Source: CAD feature listing. Evaluate the final solid. Frame: model axes, mm. A direction names the side the tool comes from. Give positions to 0.01 mm unless a question says otherwise; leave off trailing zeros. Write each loop counter-clockwise with the first axis right and the second up, starting at its lowest first coordinate (ties: lowest second). Pieces come first, ordered by that corner, then holes. Notation, with made-up numbers: (26.25, 65.25) - (30.25, 65.25) arc R31 ccw to (30.25, 101.25) - close; hole circle Ø2 at (-20.5, 35). An arc over 180 degrees is marked (long way). Answer as a JSON object with one key per item and string values. Group by question number.
from build123d import *
from build123d.topology import SkipClean

# Parameters (mm, degrees)
SKETCH1_R                = 5.5
SKETCH1_R_2              = 4.85
BOSS_EXTRUDE1_DEPTH      = 17
BOSS_EXTRUDE2_START      = -1.75
BOSS_EXTRUDE2_DEPTH      = 1.75
BOSS_EXTRUDE3_DEPTH      = 1.7
BOSS_EXTRUDE3_2_DEPTH    = 1.7
BOSS_EXTRUDE4_REACH      = 128.36
BOSS_EXTRUDE4_END_RADIUS = 4.85
SKETCH3_W                = 1.7
SKETCH3_H                = 0.6
BOSS_EXTRUDE5_START      = -9.624935
SKETCH3_2_W              = 1.7
SKETCH3_2_H              = 0.6
BOSS_EXTRUDE5_DEPTH      = 0.075066
FILLET1_R                = 0.2
BOSS_EXTRUDE6_START      = 17
SKETCH1_4_R              = 5.5
SKETCH1_4_W              = 6
SKETCH1_4_H              = 6
BOSS_EXTRUDE6_DEPTH      = 2


with BuildPart() as part:
    # Sketch1 → Boss-Extrude1 (new body)
    with BuildSketch(Plane.XZ.offset(-123.994845224)):
        with Locations(Location((0, 0, 0), (0, 0, 270))):
            Circle(SKETCH1_R)
        with Locations(Location((0, 0, 0), (0, 0, 270))):
            Circle(SKETCH1_R_2, mode=Mode.SUBTRACT)
    extrude(amount=BOSS_EXTRUDE1_DEPTH)

    # Sketch1<3> → Boss-Extrude2 (add)
    with SkipClean():  # the faces are left unmerged after this step: merging them gives an invalid solid
        with BuildSketch(Plane.XZ.offset(-123.994845224).offset(BOSS_EXTRUDE2_START)):
            with BuildLine():
                ThreePointArc((4.280924301, -3.453069233), (4.763148058, -2.74998556), (5.130919838, -1.98082347))
                Line((5.130919838, -1.98082347), (5.108754465, -1.968026376))
                Line((5.108754465, -1.968026376), (4.625228328, -1.688864385))
                Line((4.625228328, -1.688864385), (4.20023564, -2.424978467))
                Line((4.20023564, -2.424978467), (3.775232792, -3.161110148))
                Line((3.775232792, -3.161110148), (4.258758928, -3.440272139))
                Line((4.258758928, -3.440272139), (4.280924301, -3.453069233))
            make_face()
            with BuildLine():
                Line((-3.775232792, 3.161110148), (-4.258758928, 3.440272139))
                Line((-4.258758928, 3.440272139), (-4.280924301, 3.453069233))
                ThreePointArc((-4.280924301, 3.453069233), (-4.763148058, 2.74998556), (-5.130919838, 1.98082347))
                Line((-5.130919838, 1.98082347), (-5.108754465, 1.968026376))
                Line((-5.108754465, 1.968026376), (-4.625228328, 1.688864385))
                Line((-4.625228328, 1.688864385), (-4.200235262, 2.424979122))
                Line((-4.200235262, 2.424979122), (-3.775232792, 3.161110148))
            make_face()
            with BuildLine():
                Line((4.625228328, -1.688864385), (4.560219632, -1.651331859))
                ThreePointArc((4.560219632, -1.651331859), (4.397274885, -2.046087385), (4.20023564, -2.424978467))
                Line((4.20023564, -2.424978467), (4.625228328, -1.688864385))
            make_face()
            with BuildLine():
                ThreePointArc((4.20023564, -2.424978467), (3.970623818, -2.785075672), (3.710224095, -3.123577623))
                Line((3.710224095, -3.123577623), (3.775232792, -3.161110148))
                Line((3.775232792, -3.161110148), (4.20023564, -2.424978467))
            make_face()
            with BuildLine():
                ThreePointArc((-4.560219632, 1.651331859), (-4.397274725, 2.046087728), (-4.200235262, 2.424979122))
                Line((-4.200235262, 2.424979122), (-4.625228328, 1.688864385))
                Line((-4.625228328, 1.688864385), (-4.560219632, 1.651331859))
            make_face()
            with BuildLine():
                Line((-3.710224095, 3.123577623), (-3.775232792, 3.161110148))
                Line((-3.775232792, 3.161110148), (-4.200235262, 2.424979122))
                ThreePointArc((-4.200235262, 2.424979122), (-3.970623601, 2.785075982), (-3.710224095, 3.123577623))
            make_face()
        extrude(amount=BOSS_EXTRUDE2_DEPTH)



with BuildPart() as body_2:
    # Sketch2 → Boss-Extrude3 (new body)
    with BuildSketch(Plane(origin=(0.424997768, 0, 0.736122882), x_dir=(0.866026919582721, 0, -0.49999737455117027), z_dir=(0.49999737455117027, 0, 0.866026919582721))):
        Polygon((4.5, 125.144845224), (4.774934555, 125.144845224), (4.774934555, 125.744845224), align=None)
    extrude(amount=-BOSS_EXTRUDE3_DEPTH)


with BuildPart() as body_3:
    # Sketch2 → Boss-Extrude3 2 (new body)
    with BuildSketch(Plane(origin=(0.424997768, 0, 0.736122882), x_dir=(0.866026919582721, 0, -0.49999737455117027), z_dir=(0.49999737455117027, 0, 0.866026919582721))):
        Polygon((-4.5, 125.144845224), (-4.774934555, 125.744845224), (-4.774934555, 125.144845224), align=None)
    extrude(amount=-BOSS_EXTRUDE3_2_DEPTH)


with BuildPart() as part_1:
    with SkipClean():  # the faces are left unmerged after this step: merging them gives an invalid solid
        add(part.part)

        add(body_2.part)  # Boss-Extrude4 merges body 2
        # Boss-Extrude4: up to this cylinder (the profile starts inside it)
        boss_extrude4_end = Plane(origin=(0, 125.444845, 0), z_dir=(0, 1, 0)) * Cylinder(BOSS_EXTRUDE4_END_RADIUS, 267.42, mode=Mode.PRIVATE)
        # Sketch3 → Boss-Extrude4 (add, up to the surface)
        with BuildSketch(Plane(origin=(4.135221863, 0, -2.387454741), x_dir=(-0.4999973745511703, 0, -0.866026919582721), z_dir=(0.866026919582721, 0, -0.4999973745511703)), mode=Mode.PRIVATE) as boss_extrude4_sk1:
            with Locations((0, 125.444845224)):
                Rectangle(SKETCH3_W, SKETCH3_H)
        boss_extrude4_tool1 = extrude(boss_extrude4_sk1.sketch, amount=BOSS_EXTRUDE4_REACH, mode=Mode.PRIVATE) & boss_extrude4_end
        add(boss_extrude4_tool1.solids().sort_by_distance((4.135222, 125.444845, -2.387455))[0])


    with SkipClean():  # the faces are left unmerged after this step: merging them gives an invalid solid
        add(body_3.part)  # Boss-Extrude5 merges body 3
        # Sketch3<2> → Boss-Extrude5 (add)
        with BuildSketch(Plane(origin=(4.135221863, 0, -2.387454741), x_dir=(-0.4999973745511703, 0, -0.866026919582721), z_dir=(0.866026919582721, 0, -0.4999973745511703)).offset(BOSS_EXTRUDE5_START)):
            with Locations((0, 125.444845224)):
                Rectangle(SKETCH3_2_W, SKETCH3_2_H)
        extrude(amount=BOSS_EXTRUDE5_DEPTH)

    # Fillet1
    # the kernel refuses this fillet: 0.2 mm, written as the material it adds along each edge
    with BuildSketch(Plane(origin=(-4.713937761, 123.994845224, 3.70306792), x_dir=(0.49999737455195337, 0, 0.866026919582269), z_dir=(0.866026919582269, 0, -0.4999973745519534))) as fillet1_piece_1_section:
        with BuildLine():
            CenterArc((FILLET1_R, -FILLET1_R), FILLET1_R, 90, 90)
            Line((0, -FILLET1_R), (0, 0))
            Line((0, 0), (FILLET1_R, 0))
        make_face()
    fillet1_piece_1 = extrude(amount=1.083921236, mode=Mode.PRIVATE)
    fillet1_piece_1 = fillet1_piece_1 & Plane(origin=(0, 124.040443489, 0), x_dir=(0, 0, -1), z_dir=(0, 1, 0)) * Cylinder(5.5, 3, mode=Mode.PRIVATE)
    add(fillet1_piece_1)
    with BuildSketch(Plane(origin=(4.713937761, 123.994845224, -3.70306792), x_dir=(-0.49999737455261106, 0, -0.8660269195818893), z_dir=(-0.8660269195818893, 0, 0.4999973745526111))) as fillet1_piece_2_section:
        with BuildLine():
            CenterArc((FILLET1_R, -FILLET1_R), FILLET1_R, 90, 90)
            Line((0, -FILLET1_R), (0, 0))
            Line((0, 0), (FILLET1_R, 0))
        make_face()
    fillet1_piece_2 = extrude(amount=1.083921236, mode=Mode.PRIVATE)
    fillet1_piece_2 = fillet1_piece_2 & Plane(origin=(0, 124.040443489, 0), x_dir=(0, 0, -1), z_dir=(0, 1, 0)) * Cylinder(5.5, 3, mode=Mode.PRIVATE)
    add(fillet1_piece_2)
    with BuildSketch(Plane(origin=(-4.625228328, 123.994845224, 1.688864385), x_dir=(-0.49999737454985904, 0, -0.866026919583478), z_dir=(-0.8660269195834781, 0, 0.49999737454985904))) as fillet1_piece_3_section:
        with BuildLine():
            CenterArc((FILLET1_R, -FILLET1_R), FILLET1_R, 90, 90)
            Line((0, -FILLET1_R), (0, 0))
            Line((0, 0), (FILLET1_R, 0))
        make_face()
    fillet1_piece_3 = extrude(amount=1.083921236, mode=Mode.PRIVATE)
    fillet1_piece_3 = fillet1_piece_3 & Plane(origin=(0, 124.040443489, 0), x_dir=(0, 0, -1), z_dir=(0, 1, 0)) * Cylinder(5.5, 3, mode=Mode.PRIVATE)
    add(fillet1_piece_3)
    with BuildSketch(Plane(origin=(4.625228328, 123.994845224, -1.688864385), x_dir=(0.4999973745501742, 0, 0.866026919583296), z_dir=(0.8660269195832961, 0, -0.49999737455017423))) as fillet1_piece_4_section:
        with BuildLine():
            CenterArc((FILLET1_R, -FILLET1_R), FILLET1_R, 90, 90)
            Line((0, -FILLET1_R), (0, 0))
            Line((0, 0), (FILLET1_R, 0))
        make_face()
    fillet1_piece_4 = extrude(amount=1.083921236, mode=Mode.PRIVATE)
    fillet1_piece_4 = fillet1_piece_4 & Plane(origin=(0, 124.040443489, 0), x_dir=(0, 0, -1), z_dir=(0, 1, 0)) * Cylinder(5.5, 3, mode=Mode.PRIVATE)
    add(fillet1_piece_4)
    with BuildSketch(Plane(origin=(4.625228328, 123.994845224, -1.688864385), x_dir=(0.4999973745511805, 0, 0.8660269195827152), z_dir=(-0.8660269195827152, 0, 0.49999737455118054))) as fillet1_piece_5_section:
        with BuildLine():
            CenterArc((FILLET1_R, FILLET1_R), FILLET1_R, 180, 90)
            Line((0, FILLET1_R), (0, 0))
            Line((0, 0), (FILLET1_R, 0))
        make_face()
    fillet1_piece_5 = extrude(amount=0.575065445, mode=Mode.PRIVATE)
    fillet1_piece_5 = fillet1_piece_5 - Plane(origin=(0, 124.037616214, 0), x_dir=(0, 0, -1), z_dir=(0, 1, 0)) * Cylinder(4.85, 2, mode=Mode.PRIVATE)
    add(fillet1_piece_5)
    with BuildSketch(Plane(origin=(-4.625228328, 123.994845224, 1.688864385), x_dir=(-0.49999737455107873, 0, -0.8660269195827739), z_dir=(0.8660269195827739, 0, -0.49999737455107884))) as fillet1_piece_6_section:
        with BuildLine():
            CenterArc((FILLET1_R, FILLET1_R), FILLET1_R, 180, 90)
            Line((0, FILLET1_R), (0, 0))
            Line((0, 0), (FILLET1_R, 0))
        make_face()
    fillet1_piece_6 = extrude(amount=0.575065445, mode=Mode.PRIVATE)
    fillet1_piece_6 = fillet1_piece_6 - Plane(origin=(0, 124.037616214, 0), x_dir=(0, 0, -1), z_dir=(0, 1, 0)) * Cylinder(4.85, 2, mode=Mode.PRIVATE)
    add(fillet1_piece_6)
    with BuildSketch(Plane(origin=(3.277210635, 123.994845224, -2.873578935), x_dir=(-0.49999737455115034, 0, -0.8660269195827325), z_dir=(0.8660269195827326, 0, -0.49999737455115034))) as fillet1_piece_7_section:
        with BuildLine():
            CenterArc((FILLET1_R, FILLET1_R), FILLET1_R, 180, 90)
            Line((0, FILLET1_R), (0, 0))
            Line((0, 0), (FILLET1_R, 0))
        make_face()
    fillet1_piece_7 = extrude(amount=0.575065445, mode=Mode.PRIVATE)
    fillet1_piece_7 = fillet1_piece_7 - Plane(origin=(0, 124.037616214, 0), x_dir=(0, 0, -1), z_dir=(0, 1, 0)) * Cylinder(4.85, 2, mode=Mode.PRIVATE)
    add(fillet1_piece_7)
    with BuildSketch(Plane(origin=(-3.277210635, 123.994845224, 2.873578935), x_dir=(0.4999973745510395, 0, 0.8660269195827964), z_dir=(-0.8660269195827965, 0, 0.49999737455103954))) as fillet1_piece_8_section:
        with BuildLine():
            CenterArc((FILLET1_R, FILLET1_R), FILLET1_R, 180, 90)
            Line((0, FILLET1_R), (0, 0))
            Line((0, 0), (FILLET1_R, 0))
        make_face()
    fillet1_piece_8 = extrude(amount=0.575065445, mode=Mode.PRIVATE)
    fillet1_piece_8 = fillet1_piece_8 - Plane(origin=(0, 124.037616214, 0), x_dir=(0, 0, -1), z_dir=(0, 1, 0)) * Cylinder(4.85, 2, mode=Mode.PRIVATE)
    add(fillet1_piece_8)

    # Sketch1<4> → Boss-Extrude6 (add)
    with BuildSketch(Plane.XZ.offset(-123.994845224).offset(BOSS_EXTRUDE6_START)):
        with Locations(Location((0, 0, 0), (0, 0, 161.006016149))):
            Circle(SKETCH1_4_R)
        Rectangle(SKETCH1_4_W, SKETCH1_4_H, mode=Mode.SUBTRACT)
    extrude(amount=BOSS_EXTRUDE6_DEPTH)


solid = part_1.part
Q1. Section C-C on y = 106.75. Return the cut outline in (x, z).
Q2. Ray query, probe 1 along Z at (x, y) = (0, 115); probe 2 along X at (y, z) = (121, -3). Return the intervals inside material, ascending. Write a range as [from, to].
Q3. Section D-D on z = 4.5. Return the cut outline in (x, y), then the cut area to 3 significant figures.
Q4. Draft query along X for faces 6 (the flat face through (4.024, 125.449, -2.309)), 7 (the flat face through (-3, 106, 0)), 8 (the flat face through (-4.04, 125.145, 2.35)). Return one class per face: released by +X, released by -X, zero draft, split by the parting line, or undercut.
Q5. Section A-A on x = 0. Return the cut outline in (y, z).
Q6. Section B-B on z = 0. Return the cut outline in (x, y), then the cut area to 3 significant figures.
Q7. First-contact query: pin 1 Ø5 at (x, z) = (2, 2) entering from +Y; pin 2 Ø1 at (x, y) = (-0.5, 119) entering from -Z; pin 3 Ø1 at (x, y) = (-1, 105.5) entering from +Z; pin 4 Ø1 at (x, y) = (2, 108.5) entering from -Z. Flat tips, straight axial feed; report the tip coordinate or a pass-through.
Q8. Reachability of faces 1 (the flat face through (-3, 123.995, -4)), 2 (the flat face through (3, 123.995, 4)), 3 (the flat face through (0, 106, -3)), 4 (the flat face through (4, 125.745, -3)), 5 (the flat face through (4.05, 125.145, -2.33)) from +Z, -Z, +X, -X, +Y, -Y: full face, straight path, thin tool, end or side. Return the list, or none.
Taken from the geometry:
{
 "1": {"outline": "circle Ø11 at (0, 0); hole (-3, -3) - (3, -3) - (3, 3) - (-3, 3) - close"},
 "2": {"probe 1": "z = [-5.5, -4.85], [4.85, 5.5]", "probe 2": "x = [-4.61, -3.81], [3.81, 4.61]"},
 "3": {"outline": "(-3.16, 104.99) - (3.16, 104.99) - (3.16, 123.99) - (1.81, 123.99) - (1.81, 106.99) - (-1.81, 106.99) - (-1.81, 123.99) - (-3.16, 123.99) - close", "area": "58.7 mm²"},
 "4": {"face 6": "released by -X", "face 7": "undercut", "face 8": "zero draft"},
 "5": {"outline": "(104.99, -5.5) - (123.99, -5.5) - (123.99, -4.85) - (106.99, -4.85) - (106.99, -3) - (104.99, -3) - close; (104.99, 3) - (106.99, 3) - (106.99, 4.85) - (123.99, 4.85) - (123.99, 5.5) - (104.99, 5.5) - close"},
 "6": {"outline": "(-5.5, 104.99) - (-3, 104.99) - (-3, 106.99) - (-4.85, 106.99) - (-4.85, 123.99) - (-5.5, 123.99) - close; (3, 104.99) - (5.5, 104.99) - (5.5, 123.99) - (4.85, 123.99) - (4.85, 106.99) - (3, 106.99) - close", "area": "32.1 mm²"},
 "7": {"pin 1": "stops at y = 123.99", "pin 2": "stops at z = -5.5", "pin 3": "stops at z = 5.48", "pin 4": "stops at z = -5.29"},
 "8": {"face 1": "-Z, -X, +Y", "face 2": "+Z, +X, +Y", "face 3": "+Y, -Y", "face 4": "+Z, -Z, +X, -X, +Y", "face 5": "+Z, -X"}
}
